Input: part model. Units: mm. Frame: model coordinates. A direction names the side the tool comes from. Round coordinates to 2 decimals unless told otherwise and drop trailing zeros. Loops run counter-clockwise (first coordinate to the right, second up) from the corner with the lowest first, then second, coordinate; pieces in that order, holes last. Notation, with made-up numbers: M -19.5,-3.75 L 15.5,-3.75 A17 cw 15.5,10.25 Z; hole C -31,58 d11. An arc over 180 degrees is marked long. Put each result on its own line as item: value. Start each with the question number.
1) Section D-D on y = 25. Output: boundary loops of the cut face in (x, z), plus the area to 3 significant figures.
2) Pin query (flat end, axial travel): pin 1 (2.5 mm diameter, centred on x = 35, y = -25, fed in from +Z). Return the tip coordinate at first contact, or that it passes through.
3) Reachability of faces 5 (the face through (-28.289, -18.196, 1.521)), 6 (the face through (-6.7, 20.4, 0)) from +Z, -Z, +X, -X, +Y, -Y: full face, straight path, thin tool, end or side. Return the list, or none.
4) Section C-C on x = 35. Output: boundary loops of the cut face in (y, z).
5) Line query: probe 1 along Y at (x, z) = (-35, 1.4); probe 2 along Y at (x, z) = (-47.5, 1.75); probe 3 along Y at (x, z) = (-6.5, 1.2). Output: solid intervals per line, ascending.
6) Section B-B on y = 4. Output: boundary loops of the cut face in (x, z).
7) Draft query along Y for faces 1 (the face through (-53, 0, 1)), 2 (the face through (30, 0, 1)), 3 (the face through (-34.17, 23.69, 1.48)), 4 (the face through (40.43, 29.4, 1.52)). Return one class per face: +Y half, -Y half, draft (parallel to the pull), parting line (faces both ways), or undercut.
8) Section A-A on x = -12. Output: boundary loops of the cut face in (y, z).
Autodesk Inventor part; units mm, degrees
ref_plane "YZ Plane" through (0, 0, 0) normal (1, 0, 0) x (0, 1, 0)
ref_plane "XZ Plane" through (0, 0, 0) normal (0, 1, 0) x (-1, 0, 0)
ref_plane "XY Plane" through (0, 0, 0) normal (0, 0, 1) x (1, 0, 0)
sketch "Sketch1" plane through (0, 0, 0) normal (0, 0, 1) x (1, 0, 0)
  line L0 (0, 42) -> (0, -42) construction
  line L1 (-71.8, 0) -> (59.8, 0) construction
  line L2 (-39, -29) -> (39, -29) construction
  line L3 (39, -29) -> (39, 29) construction
  line L4 (39, 29) -> (-39, 29) construction
  line L5 (-39, 29) -> (-39, -29) construction
  line L6 (-39, -29) -> (39, 29) construction
  line L7 (39, -29) -> (-39, 29) construction
  line L8 (-35, -25) -> (35, -25) construction
  line L9 (35, -25) -> (35, 25) construction
  line L10 (35, 25) -> (-35, 25) construction
  line L11 (-35, 25) -> (-35, -25) construction
  line L12 (-35, -25) -> (35, 25) construction
  line L13 (35, -25) -> (-35, 25) construction
  circle A0 centre (-35, 25) radius 1.55
  circle A1 centre (-35, -25) radius 1.55
  circle A2 centre (35, -25) radius 1.55
  circle A3 centre (35, 25) radius 1.55
  line L14 (-53, 30) -> (41, 30)
  line L15 (41, 30) -> (41, -30)
  line L16 (41, -30) -> (-53, -30)
  line L17 (-53, -30) -> (-53, 30)
  line L18 (-30, -20) -> (30, -20)
  line L19 (30, -20) -> (30, 20)
  line L20 (30, 20) -> (-30, 20)
  line L21 (-30, 20) -> (-30, -20)
  line L22 (-30, -20) -> (30, 20) construction
  line L23 (30, -20) -> (-30, 20) construction
  circle A4 centre (-47.5, 20) radius 2.55
  circle A5 centre (-47.5, -20) radius 2.55
  point P0 (0, 0)
  point P1 (-53, 0)
  point P2 (-39, 0)
  dimension "d4" = 58
  dimension "d5" = 78
  dimension "d6" = 4
  dimension "d7" = 50
  dimension "d8" = 3.1
  dimension "d9" = 14
  dimension "d10" = 60
  dimension "d12" = 40
  dimension "d13" = 60
  dimension "d16" = 2
  dimension "d17" = 5.1
  dimension "d18" = 20
  dimension "d19" = 5.5
  dimension "d20" = 20
extrude "Extrusion3" add sketch "Sketch1" along normal blind 3
fillet "Fillet1" radius 6 4 edges at (-30, 20, 1.5) (-30, -20, 1.5) (30, -20, 1.5) (30, 20, 1.5)
fillet "Fillet2" radius 2 4 edges at (41, 30, 1.5) (-53, 30, 1.5) (-53, -30, 1.5) (41, -30, 1.5)
properties part number "PCB plate" material "ALMg4,5Mn-5083-(D54S)"
Geometry results:
1. outline: M -53,0 L -36.55,0 L -36.55,3 L -53,3 Z; M -33.45,0 L 33.45,0 L 33.45,3 L -33.45,3 Z; M 36.55,0 L 41,0 L 41,3 L 36.55,3 Z
1. area: 263 mm²
2. pin 1: passes through
3. face 5: +Z, -Z
3. face 6: -Z, +X, -X, +Y, -Y
4. outline: M -30,0 L -26.55,0 L -26.55,3 L -30,3 Z; M -23.45,0 L 23.45,0 L 23.45,3 L -23.45,3 Z; M 26.55,0 L 30,0 L 30,3 L 26.55,3 Z
5. probe 1: y = -30 to -26.55, -23.45 to 23.45, 26.55 to 30
5. probe 2: y = -30 to -22.55, -17.45 to 17.45, 22.55 to 30
5. probe 3: y = -30 to -20, 20 to 30
6. outline: M -53,0 L -30,0 L -30,3 L -53,3 Z; M 30,0 L 41,0 L 41,3 L 30,3 Z
7. face 1: draft
7. face 2: undercut
7. face 3: undercut
7. face 4: +Y half
8. outline: M -30,0 L -20,0 L -20,3 L -30,3 Z; M 20,0 L 30,0 L 30,3 L 20,3 Z
